Geometry: final body of the model. Coordinates: model frame, mm. A direction names the side the tool comes from. Round coordinates to 2 decimals unless told otherwise and drop trailing zeros. Loops run counter-clockwise (first coordinate to the right, second up) from the corner with the lowest first, then second, coordinate; pieces in that order, holes last. Notation, with made-up numbers: M 32.25,30 L 88.25,30 A28 cw 88.25,55 Z; hole C 46,60.5 d3. An arc over 180 degrees is marked long. Write each question's results on one line, items separated by ' | '.
```python
from build123d import *

# Parameters (mm, degrees)
SKETCH2_R          = 5
CUT_EXTRUDE1_DEPTH = 20
CUT_EXTRUDE2_DEPTH = 5


with BuildPart() as part:
    # Sketch1 → Base-Revolve (revolve)
    with BuildSketch(Plane.XY, mode=Mode.PRIVATE) as base_revolve_sk:
        with BuildLine():
            Line((0, -89), (5, -89))
            Line((5, -89), (7.5, -80))
            Line((7.5, -80), (7.5, 58.009618943))
            ThreePointArc((7.5, 58.009618943), (14.488887394, 74.882285677), (0, 86))
            Line((0, 86), (0, -89))
        make_face()
    revolve(base_revolve_sk.sketch.rotate(Axis((0, 111, 0), (0, -1, 0)), 180), axis=Axis((0, 111, 0), (0, -1, 0)))

    # Sketch2 → Cut-Extrude1 (cut, symmetric)
    with BuildSketch(Plane.XY):
        with Locations(Location((0, 70, 0), (0, 0, 236.639256329))):
            Circle(SKETCH2_R)
    extrude(amount=CUT_EXTRUDE1_DEPTH, both=True, mode=Mode.SUBTRACT)

    # Sketch3 → Cut-Extrude2 (cut, symmetric)
    with BuildSketch(Plane.XY):
        with BuildLine():
            Line((40, 110), (-40, 110))
            Line((-40, 110), (-8.209705454, 64.290294546))
            ThreePointArc((-8.209705454, 64.290294546), (0, 60), (8.209705454, 64.290294546))
            Line((8.209705454, 64.290294546), (40, 110))
        make_face()
    extrude(amount=CUT_EXTRUDE2_DEPTH, both=True, mode=Mode.SUBTRACT)


solid = part.part
```
1. Section D-D (y = 3.5). Output: boundary loops of the cut face in (x, z).
Answer key:
outline: C 0,0 d15
2. Section B-B (y = 70). Output: boundary loops of the cut face in (x, z), then the cut area to 3 significant figures.
Answer key:
outline: M -12.18,-5 L -12.18,5 L -5,5 L -5,14.11 A14.97 ccw -5,-14.11 L -5,-5 Z; M 5,-14.11 A14.97 ccw 5,14.11 L 5,5 L 12.18,5 L 12.18,-5 L 5,-5 Z | area: 266 mm²
3. Ray query, probe 1 along X at (y, z) = (70, -10.5); probe 2 along X at (y, z) = (70, 9.5); probe 3 along Y at (x, z) = (0, 12). Return the intervals inside material, ascending.
Answer key:
probe 1: x = -10.67 to -5, 5 to 10.67 | probe 2: x = -11.57 to -5, 5 to 11.57 | probe 3: y = 62 to 65, 75 to 80
4. Section A-A (z = 0). Output: boundary loops of the cut face in (x, y).
Answer key:
outline: M -14.75,73.7 A15 ccw -7.5,58.01 L -7.5,-80 L -5,-89 L 5,-89 L 7.5,-80 L 7.5,58.01 A15 ccw 14.75,73.7 L 8.21,64.29 A10 cw -8.21,64.29 Z
5. Access query for faces 1 (the face through (11.436, 68.93, 0.07)), 2 (the face through (-4.032, -10.029, -6.324)), 3 (the face through (0, -89, 0)). Directions: +Z, -Z, +X, -X, +Y, -Y. A direction counts if a zero-diameter tool reaches every point of the face in a straight line with its end or side. Return the directions, or none.
Answer key:
face 1: +Y | face 2: -Y | face 3: +Z, -Z, +X, -X, -Y
6. Pin query (flat end, axial travel): P1, Ø7.5, axis at x = 3.5, y = 72.5, coming from the -Z side; P2, Ø5, axis at x = -4.5, y = 4.5, coming from the +Z side; P3, Ø6, axis at y = -39, z = 4.5, coming from the -X side; P4, Ø9, axis at x = 0, y = 70, coming from the -Z side. Return the tip coordinate at first contact, or that it passes through.
Answer key:
P1: stops at z = -14.45 | P2: stops at z = 7.23 | P3: stops at x = -7.35 | P4: passes through
7. Section C-C (x = 0). Output: boundary loops of the cut face in (y, z).
Answer key:
outline: M -89,-5 L -80,-7.5 L 58.01,-7.5 A15 ccw 65,-13.75 L 65,-5 L 60,-5 L 60,5 L 65,5 L 65,13.75 A15 ccw 58.01,7.5 L -80,7.5 L -89,5 Z; M 75,-14.46 A15 ccw 85.14,-5 L 75,-5 Z; M 75,5 L 85.14,5 A15 ccw 75,14.46 Z
8. Draft query along Z for faces 4 (the face through (0, 75, -10)), 5 (the face through (-5.448, -86.437, -1.716)), 6 (the face through (0, 60, 0)). Return one class per face: pulls with the +Z half, pulls with the -Z half, needs draft (parallel to the pull), parting line crosses it, or undercut.
Answer key:
face 4: needs draft | face 5: parting line crosses it | face 6: undercut
